The figure shows three views and two pictorial views of one solid part (mm, origin at its lowest corner). Answer the questions. A direction names the side the tool comes from. Coordinates: 2 decimals unless noted, no trailing zeros. Loops run counter-clockwise (first coordinate to the right, second up) from the corner with the lowest first, then second, coordinate; pieces in that order, holes last. Notation, with made-up numbers: (-18, -29) -> (36, -29) arc R14 cw to (36, -20) -> close; hole circle Ø7 at (52.25, 27.5). An arc over 180 degrees is marked (long way). Answer as a JSON object with one key per item and string values. Group by question number.
1) Which of the six approach directions +Z, -Z, +X, -X, +Y, -Y give full straight-line access (tool end or side, diameter ignored) to the marked faces 1 and 2?
2) Flat-ended cylindrical pins translate along their axes: P1, Ø6, axis at x = 13.5, z = 29.5, coming from the -Y side; P2, Ø12, axis at x = 31.5, y = 4, coming from the -Z side; P3, Ø12, axis at x = 8.5, y = 3.5, coming from the +Z side; P4, Ø10, axis at y = 10, z = 98.5, coming from the -X side. Find the tip coordinate at first contact, or state that the pin passes through.
3) Section A-A, the plane x = 19 is taken. Give the vertices of the cut face in (y, z), plus the area to 3 significant figures.
4) Section C-C, the plane z = 103 is taken. Give the vertices of the cut face in (x, y), plus the area to 3 significant figures.
5) Section D-D, the plane y = 6 is taken. Give the vertices of the cut face in (x, z).
6) Section B-B, the plane y = 15 is taken. Give the vertices of the cut face in (x, z), plus the area to 3 significant figures.
7) Consider probe 1 along Z at (x, y) = (26.5, 15.5); probe 2 along Y at (x, z) = (19.5, 109). Determine where each line is inside the solid, lowest interval first. Write a range as [from, to].
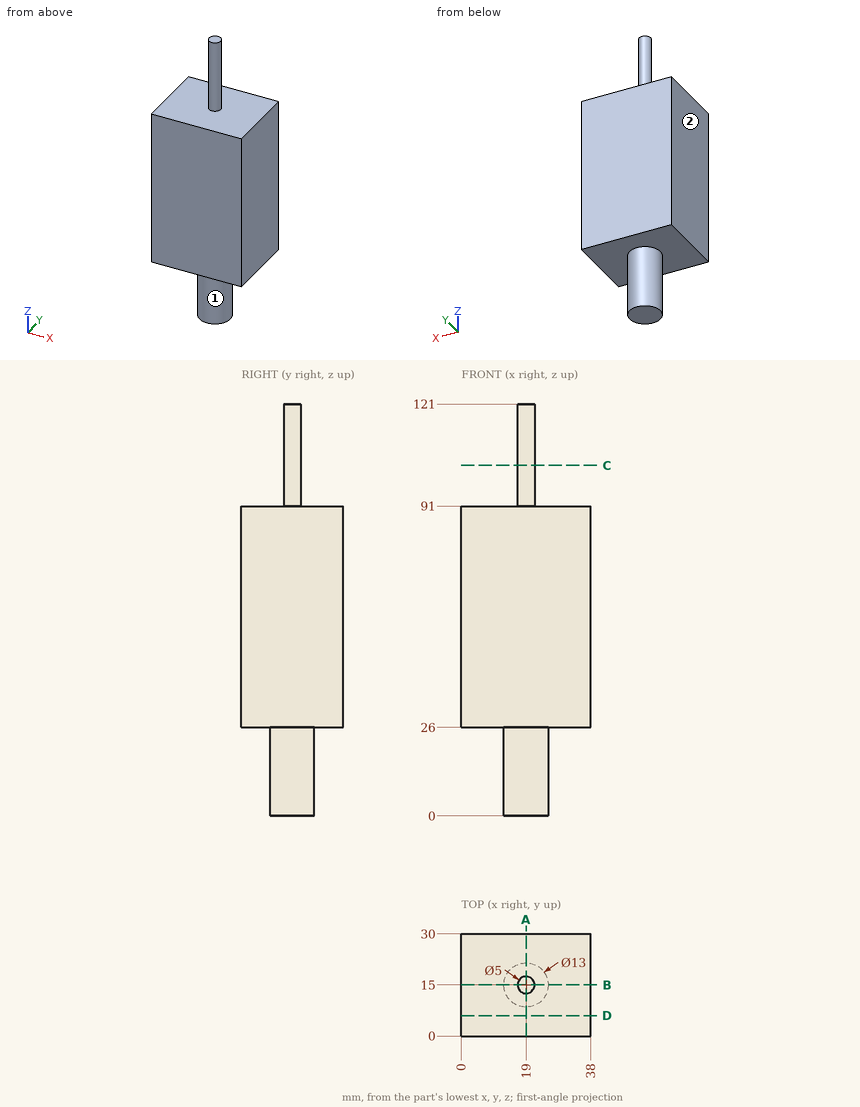
Determined:
{
 "1": {"face 1": "-Z", "face 2": "+Z, -Z, -X, +Y, -Y"},
 "2": {"P1": "y = 0", "P2": "z = 26", "P3": "z = 91", "P4": "x = 16.5"},
 "3": {"outline": "(0, 26) -> (8.5, 26) -> (8.5, 0) -> (21.5, 0) -> (21.5, 26) -> (30, 26) -> (30, 91) -> (17.5, 91) -> (17.5, 121) -> (12.5, 121) -> (12.5, 91) -> (0, 91) -> close", "area": "2,440 mm²"},
 "4": {"outline": "circle Ø5 at (19, 15)", "area": "19.6 mm²"},
 "5": {"outline": "(0, 26) -> (38, 26) -> (38, 91) -> (0, 91) -> close"},
 "6": {"outline": "(0, 26) -> (12.5, 26) -> (12.5, 0) -> (25.5, 0) -> (25.5, 26) -> (38, 26) -> (38, 91) -> (21.5, 91) -> (21.5, 121) -> (16.5, 121) -> (16.5, 91) -> (0, 91) -> close", "area": "2,960 mm²"},
 "7": {"probe 1": "[26, 91]", "probe 2": "[12.55, 17.45]"}
}
